Geometry: final body of the model. Coordinates: model frame, mm. A direction names the side the tool comes from. Coordinates: 2 decimals unless noted, no trailing zeros. Order: outer loops, then holes, each group sorted by start corner. A loop starts at its lowest first (then second) coordinate and runs counter-clockwise, first axis right, second up. Notation, with made-up numbers: M 11.25,-21 L 48.25,-21 A22 cw 48.25,2 Z; hole C -36,50.25 d9. An arc over 180 degrees is marked long. Use CSV: the item, a comma, the result in double quotes. Start each with the question number.
1. Section query A-A on x = -625. Return the cut outline in (y, z), and give its area (3 significant figures).
2. Material intervals for line 1 (Y direction, x = -620, z = 202); line 2 (Z direction, x = -1016, y = 485); line 3 (Z direction, x = -907, y = 685), sorted ascending.
3. First-contact query: P1, Ø2, axis at x = -428.5, z = 254.5, coming from the -Y side; P2, Ø5, axis at x = -890.5, z = 293, coming from the +Y side; P3, Ø8, axis at x = -268, z = 392, coming from the -Y side. Flat tips, straight axial feed; report the tip coordinate or a pass-through.
4. Section query D-D on x = -850. Return the cut outline in (y, z), and give its area (3 significant figures).
5. Set-up query: faces 1 (the flat face through (-912, 1167, 40)), 2 (the flat face through (-626, 801, 450)). Return all of +Z, -Z, +X, -X, +Y, -Y with unobstructed straight access to the full face (end or side cutting, diameter ignored); none if empty.
6. Section query B-B on y = 800. Return the cut outline in (x, z), and give its area (3 significant figures).
7. Section query C-C on z = 415. Return the cut outline in (x, y).
from build123d import *

# Parameters (mm, degrees)
ESQUISSE1_W        = 1250
ESQUISSE1_H        = 1600
BOSS_EXTRU_1_DEPTH = 40
ESQUISSE2_R        = 440
BOSS_EXTRU_2_DEPTH = 400
ESQUISSE3_R        = 50
BOSS_EXTRU_3_DEPTH = 10


with BuildPart() as part:
    # Esquisse1 → Boss.-Extru.1 (new body)
    with BuildSketch(Plane.XY):
        with Locations((-625, 800)):
            Rectangle(ESQUISSE1_W, ESQUISSE1_H)
    extrude(amount=BOSS_EXTRU_1_DEPTH)

    # Esquisse2 → Boss.-Extru.2 (add)
    with BuildSketch(Plane.XY.offset(40)):
        with Locations((-625, 800)):
            Circle(ESQUISSE2_R)
    extrude(amount=BOSS_EXTRU_2_DEPTH)

    # Esquisse3 → Boss.-Extru.3 (add)
    with BuildSketch(Plane.XY.offset(440)):
        with Locations((-625, 800)):
            Circle(ESQUISSE3_R)
    extrude(amount=BOSS_EXTRU_3_DEPTH)


solid = part.part
Results list:
1,outline,"M 0,0 L 1600,0 L 1600,40 L 1240,40 L 1240,440 L 850,440 L 850,450 L 750,450 L 750,440 L 360,440 L 360,40 L 0,40 Z"
1,area,"417,000 mm²"
2,line 1,"y = 360.03 to 1239.97"
2,line 2,"z = 0 to 40"
2,line 3,"z = 0 to 440"
3,P1,"stops at y = 405.82"
3,P2,"stops at y = 1152.75"
3,P3,"stops at y = 537.34"
4,outline,"M 0,0 L 1600,0 L 1600,40 L 1178.12,40 L 1178.12,440 L 421.88,440 L 421.88,40 L 0,40 Z"
4,area,"366,000 mm²"
5,face 1,"+Z"
5,face 2,"+Z, +X, -X, +Y, -Y"
6,outline,"M -1250,0 L 0,0 L 0,40 L -185,40 L -185,440 L -575,440 L -575,450 L -675,450 L -675,440 L -1065,440 L -1065,40 L -1250,40 Z"
6,area,"403,000 mm²"
7,outline,"C -625,800 d880"
